The model under review builds one solid part; all positions refer to its coordinate system, in mm. Face numbers are marked on the shaded views. A direction names the side the tool comes from. Coordinates: 2 decimals unless noted, no trailing zeros. Write each loop counter-clockwise with the first axis right and the second up, starting at its lowest first coordinate (ties: lowest second). Pieces come first, ordered by that corner, then holes.
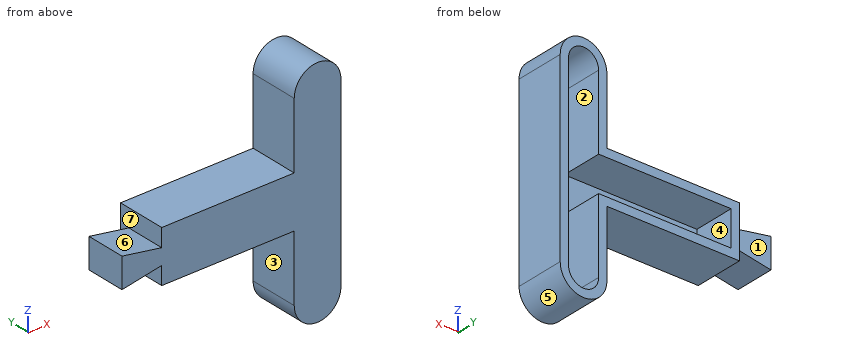
```python
from build123d import *

# Parameters (mm, degrees)
BOSS_EXTRUDE1_DEPTH = 38.1
CUT_EXTRUDE10_DEPTH = 7.62
SHELL2_START        = 6.35
SHELL2_DEPTH        = 31.75
SHELL2_2_DEPTH      = 17.78


# Read off the part's stored shape, not the designer's step: Shell2
with BuildPart() as part:
    # Sketch1 → Boss-Extrude1 (new body)
    with BuildSketch(Plane(origin=(0, 0, 0), x_dir=(1, 0, 0), z_dir=(0, 1, 0))):
        with BuildLine():
            Line((0, 11.43), (0, -11.43))
            Line((0, -11.43), (30.48, -6.055553628))
            Line((30.48, -6.055553628), (30.48, -19.771553628))
            Line((30.48, -19.771553628), (132.08, -19.771553628))
            Line((132.08, -19.771553628), (132.08, -70.571553628))
            ThreePointArc((132.08, -70.571553628), (149.987, -88.478553628), (167.894, -70.571553628))
            Line((167.894, -70.571553628), (167.894, 70.571553628))
            ThreePointArc((167.894, 70.571553628), (149.987, 88.478553628), (132.08, 70.571553628))
            Line((132.08, 70.571553628), (132.08, 19.771553628))
            Line((132.08, 19.771553628), (30.48, 19.771553628))
            Line((30.48, 19.771553628), (30.48, 6.055553628))
            Line((30.48, 6.055553628), (0, 11.43))
        make_face()
    extrude(amount=BOSS_EXTRUDE1_DEPTH)

    # Sketch5 → Cut-Extrude10 (cut)
    with BuildSketch(Plane(origin=(0, 38.1, 0), x_dir=(1, 0, 0), z_dir=(0, 1, 0))):
        Polygon((0, -11.43), (0, 11.43), (0.205611809, 11.576348711), (30.48, 6.055553628), (30.48, -6.055553628), align=None)
    extrude(amount=-CUT_EXTRUDE10_DEPTH, mode=Mode.SUBTRACT)

    # Shell2 outline → Shell2 (cut)
    with BuildSketch(Plane(origin=(0, 0, 0), x_dir=(1, 0, 0), z_dir=(0, 1, 0)).offset(SHELL2_START)):
        with BuildLine():
            Line((36.83, 13.421553628), (36.83, -13.421553628))
            Line((36.83, -13.421553628), (138.43, -13.421553628))
            Line((138.43, -13.421553628), (138.43, -70.571553628))
            ThreePointArc((138.43, -70.571553628), (149.987, -82.128553628), (161.544, -70.571553628))
            Line((161.544, -70.571553628), (161.544, 70.571553628))
            ThreePointArc((161.544, 70.571553628), (149.987, 82.128553628), (138.43, 70.571553628))
            Line((138.43, 70.571553628), (138.43, 13.421553628))
            Line((138.43, 13.421553628), (36.83, 13.421553628))
        make_face()
    extrude(amount=SHELL2_DEPTH, mode=Mode.SUBTRACT)

    # Shell2 2 outline → Shell2 2 (cut)
    with BuildSketch(Plane(origin=(0, 0, 0), x_dir=(1, 0, 0), z_dir=(0, 1, 0)).offset(SHELL2_START)):
        Polygon((28.25455863, 0), (6.35, 3.862364687), (6.35, -3.862364687), align=None)
    extrude(amount=SHELL2_2_DEPTH, mode=Mode.SUBTRACT)


solid = part.part
```
Item 1: To check wall thickness, follow line 1 along Z through (x, y) = (41, 14); line 2 along Z through (x, y) = (149.5, 27); line 3 along X through (y, z) = (8.5, -65.5). State the ranges of each line that lie inside material, in increasing order.
Solved:
line 1: z = -19.77 to -13.42, 13.42 to 19.77
line 2: z = -88.47 to -82.12, 82.12 to 88.47
line 3: x = 132.08 to 138.43, 161.54 to 167.89
Item 2: For pin 1 (2 mm diameter, centred on x = 145, z = -63.5, fed in from +Y); pin 2 (12 mm diameter, centred on x = 102.5, z = -16, fed in from -Y); pin 3 (5 mm diameter, centred on y = 31.5, z = 25, fed in from -X); pin 4 (8.5 mm diameter, centred on x = 20, z = -1, fed in from +Y), all flat-tipped, find the tip position at first contact; note any pin that passes through.
Solved:
pin 1: stops at y = 6.35
pin 2: stops at y = 0
pin 3: stops at x = 132.08
pin 4: stops at y = 30.48
Item 3: Take a section at B-B, the plane x = 62. Write out the cut boundary in (y, z), plus the area to 3 significant figures.
Solved:
outline: (0, -19.77) - (38.1, -19.77) - (38.1, -13.42) - (6.35, -13.42) - (6.35, 13.42) - (38.1, 13.42) - (38.1, 19.77) - (0, 19.77) - close
area: 654 mm2
Item 4: Take a section at D-D, the plane y = 21. Write out the cut boundary in (x, z).
Solved:
outline: (0, -11.43) - (30.48, -6.06) - (30.48, -19.77) - (132.08, -19.77) - (132.08, -70.57) arc R17.91 ccw to (167.89, -70.57) - (167.89, 70.57) arc R17.91 ccw to (132.08, 70.57) - (132.08, 19.77) - (30.48, 19.77) - (30.48, 6.06) - (0, 11.43) - close; hole (6.35, -3.86) - (28.25, 0) - (6.35, 3.86) - close; hole (36.83, -13.42) - (138.43, -13.42) - (138.43, -70.57) arc R11.56 ccw to (161.54, -70.57) - (161.54, 70.57) arc R11.56 ccw to (138.43, 70.57) - (138.43, 13.42) - (36.83, 13.42) - close
Item 5: Take a section at C-C, the plane z = 9. Write out the cut boundary in (x, y), plus the area to 3 significant figures.
Solved:
outline: (0, 0) - (13.78, 0) - (13.78, 30.48) - (0, 30.48) - close; (30.48, 0) - (167.89, 0) - (167.89, 38.1) - (161.54, 38.1) - (161.54, 6.35) - (36.83, 6.35) - (36.83, 38.1) - (30.48, 38.1) - close
area: 1,700 mm2
Item 6: Mouldability with a two-part tool opening along Z and no side actions: class the marked faces 4, 5, 6 and 7 as pulls with the +Z half, pulls with the -Z half, needs draft (parallel to the pull), parting line crosses it, or undercut.
Solved:
face 4: undercut
face 5: pulls with the -Z half
face 6: pulls with the +Z half
face 7: needs draft
Item 7: Machinability: for the marked faces 1, 2 and 3, which of the approach directions +Z, -Z, +X, -X, +Y, -Y give a long, thin tool a straight path to every point of the face, cutting with its end or side? Answer none if there is none.
Solved:
face 1: +Z, -Z, -X, +Y
face 2: +Y
face 3: -Z, -X, +Y, -Y
Item 8: Take a section at A-A, the plane y = 35.5. Write out the cut boundary in (x, z).
Solved:
outline: (30.48, -19.77) - (132.08, -19.77) - (132.08, -70.57) arc R17.91 ccw to (167.89, -70.57) - (167.89, 70.57) arc R17.91 ccw to (132.08, 70.57) - (132.08, 19.77) - (30.48, 19.77) - close; hole (36.83, -13.42) - (138.43, -13.42) - (138.43, -70.57) arc R11.56 ccw to (161.54, -70.57) - (161.54, 70.57) arc R11.56 ccw to (138.43, 70.57) - (138.43, 13.42) - (36.83, 13.42) - close
